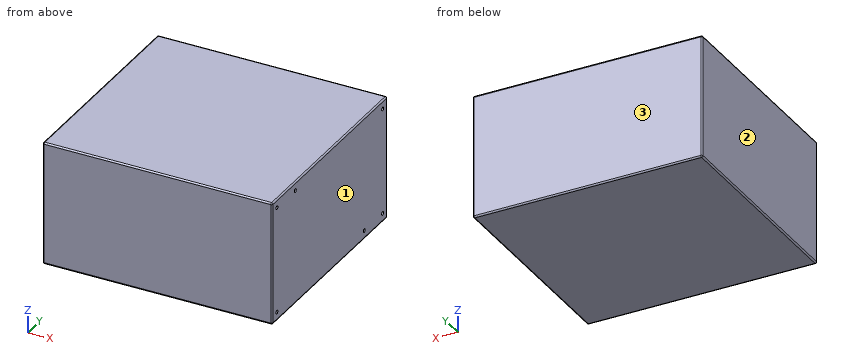
from build123d import *

# Parameters (mm, degrees)
F0_W     = 160
F0_H     = 150
F1_DEPTH = 86
F2_R     = 1.25
F3_DEPTH = 6
F4_R     = 1


with BuildPart() as f1:
    # F0 (on Top) → F1 (new body)
    with BuildSketch(Plane.XY):
        with Locations((80, 75)):
            Rectangle(F0_W, F0_H)
    extrude(amount=F1_DEPTH)

    # F2 (on face) → F3 (cut)
    with BuildSketch(Plane.YZ.offset(160)):
        with Locations((6, 80)):
            Circle(F2_R)
        with Locations((30, 80)):
            Circle(F2_R)
        with Locations((144, 80)):
            Circle(F2_R)
        with Locations((144, 6)):
            Circle(F2_R)
        with Locations((6, 6)):
            Circle(F2_R)
        with Locations((120, 6)):
            Circle(F2_R)
    extrude(amount=-F3_DEPTH, mode=Mode.SUBTRACT)

    # F4
    f4_edges = [f1.edges().sort_by_distance(p)[0] for p in [
        (160, 75, 86),
        (80, 0, 86),
        (160, 0, 43),
        (80, 150, 86),
        (0, 75, 86),
        (80, 0, 0),
        (0, 0, 43),
        (160, 75, 0),
        (160, 150, 43),
        (80, 150, 0),
        (0, 75, 0),
        (0, 150, 43),
    ]]
    fillet(f4_edges, radius=F4_R)


solid = f1.part
Can you work these out from the model? Positions are in its coordinate system, mm. Face numbers are marked on the shaded views. Round coordinates to 2 decimals unless told otherwise and drop trailing zeros. Answer in a Markdown table with one row per item. Add a question column.
Q1. I need wall thicknesses on L1, parallel to Z at x = 157.1, y = 144; L2, parallel to Y at x = 157, z = 80; L3, parallel to X at y = 120, z = 7. Which ranges of each line are inside material? Lowest first, please.
Q2. We'd pull the mould along X, two halves only. Please class the marked faces 1, 2 and 3: pulls with the +X half, pulls with the -X half, needs draft (parallel to the pull), parting line crosses it, or undercut.
Q3. For pin 1 Ø0.8 at (y, z) = (144, 6) entering from +X, with a flat end and sliding along its axis, tell me the tip position at first contact or that it passes through.
A:
| question | item | result |
|---|---|---|
| 1 | L1 | 0 to 4.75, 7.25 to 78.75, 81.25 to 86 |
| 1 | L2 | 0 to 4.75, 7.25 to 28.75, 31.25 to 142.75, 145.25 to 150 |
| 1 | L3 | 0 to 154 |
| 2 | face 1 | pulls with the +X half |
| 2 | face 2 | pulls with the -X half |
| 2 | face 3 | needs draft |
| 3 | pin 1 | x = 154 |
